from build123d import *

# Parameters (mm, degrees)
EXTRUDE_1_DEPTH     = 40
SKETCH_8_R          = 2
CUT_EXTRUDE_1_DEPTH = 50
SKETCH_9_R          = 2
CUT_EXTRUDE_2_DEPTH = 30
SKETCH_10_R         = 4.000599978
SKETCH_10_R_2       = 4
CUT_EXTRUDE_3_DEPTH = 10
CUT_EXTRUDE_START   = -10
SKETCH_11_R         = 4
CUT_EXTRUDE_4_DEPTH = 10
SKETCH_12_R         = 2
CUT_EXTRUDE_5_DEPTH = 40


with BuildPart() as part:
    # Эскиз1 → Бобышка-Вытянуть1 (new body)
    with BuildSketch(Plane.XY):
        with BuildLine():
            Line((0, 0), (130, 0))
            Line((130, 0), (130, 40))
            Line((130, 40), (0, 40))
            Line((0, 40), (0, 21))
            Line((0, 21), (12.566965626, 21))
            ThreePointArc((12.566965626, 21), (27.5, 20), (12.566965626, 19))
            Line((12.566965626, 19), (0, 19))
            Line((0, 19), (0, 0))
        make_face()
        with BuildLine():
            Line((67.433034374, 21), (77.433034374, 21))
            Line((77.433034374, 21), (77.433034374, 19))
            Line((77.433034374, 19), (67.433034374, 19))
            ThreePointArc((67.433034374, 19), (60, 12.5), (52.566965626, 19))
            Line((52.566965626, 19), (37.566965626, 19))
            Line((37.566965626, 19), (37.566965626, 21))
            Line((37.566965626, 21), (52.566965626, 21))
            ThreePointArc((52.566965626, 21), (60, 27.5), (67.433034374, 21))
        make_face(mode=Mode.SUBTRACT)
    extrude(amount=EXTRUDE_1_DEPTH)

    # Эскиз8 → Вырез-Вытянуть1 (cut)
    with BuildSketch(Plane.XZ):
        with Locations(Location((8, 30, 0), (0, 0, 270))):
            Circle(SKETCH_8_R)
        with Locations(Location((8, 10, 0), (0, 0, 270))):
            Circle(SKETCH_8_R)
        with Locations(Location((48, 30, 0), (0, 0, 270))):
            Circle(SKETCH_8_R)
        with Locations(Location((48, 10, 0), (0, 0, 270))):
            Circle(SKETCH_8_R)
    extrude(amount=-CUT_EXTRUDE_1_DEPTH, mode=Mode.SUBTRACT)

    # Эскиз9 → Вырез-Вытянуть2 (cut)
    with BuildSketch(Plane(origin=(130, 0, 0), x_dir=(0, 0, -1), z_dir=(1, 0, 0))):
        with Locations((-32, 35)):
            Circle(SKETCH_9_R)
        with Locations((-8, 35)):
            Circle(SKETCH_9_R)
        with Locations((-8, 5)):
            Circle(SKETCH_9_R)
        with Locations((-32, 5)):
            Circle(SKETCH_9_R)
    extrude(amount=-CUT_EXTRUDE_2_DEPTH, mode=Mode.SUBTRACT)

    # Эскиз10 → Вырез-Вытянуть3 (cut)
    with BuildSketch(Plane(origin=(0, 40, 0), x_dir=(1, 0, 0), z_dir=(0, 1, 0))):
        with Locations(Location((110, -8, 0), (0, 0, 270))):
            Circle(SKETCH_10_R)
        with Locations(Location((110, -32, 0), (0, 0, 270))):
            Circle(SKETCH_10_R_2)
    extrude(amount=-CUT_EXTRUDE_3_DEPTH, mode=Mode.SUBTRACT)

    # Эскиз11 → Вырез-Вытянуть4 (cut)
    with BuildSketch(Plane.XZ.offset(CUT_EXTRUDE_START)):
        with Locations(Location((110, 32, 0), (0, 0, 90))):
            Circle(SKETCH_11_R)
        with Locations(Location((110, 8, 0), (0, 0, 270))):
            Circle(SKETCH_11_R)
    extrude(amount=CUT_EXTRUDE_4_DEPTH, mode=Mode.SUBTRACT)

    # Эскиз12 → Вырез-Вытянуть5 (cut)
    with BuildSketch(Plane.XZ):
        with Locations(Location((72, 19, 0), (0, 0, 270))):
            Circle(SKETCH_12_R)
    extrude(amount=-CUT_EXTRUDE_5_DEPTH, mode=Mode.SUBTRACT)


solid = part.part
Could you check a few things on this model? Use its own coordinates, in mm. A direction names the side the tool comes from. Coordinates: 2 decimals unless noted, no trailing zeros. Write each loop counter-clockwise with the first axis right and the second up, starting at its lowest first coordinate (ties: lowest second). Pieces come first, ordered by that corner, then holes. Notation, with made-up numbers: M -35.75,-34.5 L 11.25,-34.5 A28 ccw 11.25,-3.5 Z; hole C 39.25,44 d7. An arc over 180 degrees is marked long. One line per question, with ' | ' between items.
1) I need wall thicknesses on probe 1 along Z at (x, y) = (101.75, 5); probe 2 along Y at (x, z) = (102.5, 8); probe 3 along Y at (x, z) = (19.5, 24.5). Which ranges of each line are inside material? Lowest first, please. Write a range as [from, to].
Checks:
probe 1: [0, 6], [10, 30], [34, 40] | probe 2: [0, 3], [7, 33], [37, 40] | probe 3: [0, 12.52], [27.48, 40]
2) Imagine slicing it at A-A, the plane x = 72. Write out the boundary of the cut face in (y, z), and give its area (3 significant figures).
Checks:
outline: M 0,0 L 19,0 L 19,17 L 0,17 Z; M 0,21 L 19,21 L 19,40 L 0,40 Z; M 21,0 L 40,0 L 40,17 L 21,17 Z; M 21,21 L 40,21 L 40,40 L 21,40 Z | area: 1,370 mm²
3) Imagine slicing it at D-D, the plane x = 48. Write out the boundary of the cut face in (y, z).
Checks:
outline: M 0,0 L 19,0 L 19,8 L 0,8 Z; M 0,12 L 19,12 L 19,28 L 0,28 Z; M 0,32 L 19,32 L 19,40 L 0,40 Z; M 21,0 L 40,0 L 40,8 L 21,8 Z; M 21,12 L 40,12 L 40,28 L 21,28 Z; M 21,32 L 40,32 L 40,40 L 21,40 Z
4) Imagine slicing it at C-C, the plane z = 37.5. Write out the boundary of the cut face in (x, y), and give its area (3 significant figures).
Checks:
outline: M 0,0 L 130,0 L 130,40 L 0,40 L 0,21 L 12.57,21 A7.5 cw long 12.57,19 L 0,19 Z; hole M 37.57,19 L 52.57,19 A7.5 ccw 67.43,19 L 77.43,19 L 77.43,21 L 67.43,21 A7.5 ccw 52.57,21 L 37.57,21 Z | area: 4,770 mm²
5) For pin 1 Ø2.5 at (x, z) = (111, 9.5) entering from +Y; pin 2 Ø1.2 at (y, z) = (34.5, 7.5) entering from +X; pin 3 Ø3.5 at (x, z) = (48, 30) entering from +Y, each with a flat end and sliding along its axis, tell me the tip position at first contact or that it passes through.
Checks:
pin 1: y = 30 | pin 2: x = 100 | pin 3: through
6) For faces 1 (the face through (10, 30, 10)), 2 (the face through (100, 5, 8)), 3 (the face through (113.373, 5.07, 5.85)), 4 (the face through (110, 30, 8)), 5 (the face through (75, 21, 20)), which set-ups out of +Z, -Z, +X, -X, +Y, -Y let a thin tool reach every point of the face, with its end or its side?
Checks:
face 1: +Y, -Y | face 2: +X | face 3: -Y | face 4: +Y | face 5: +Z, -Z
7) If we mould it in two halves opening along Y, with no side actions, what happens to faces 6 (the face through (100, 35, 8)), 7 (the face through (8.601, 9.367, 28.092)), 8 (the face through (75, 19, 20)), 9 (the face through (110, 10, 8))? For each: released by +Y, released by -Y, zero draft, split by the parting line, or undercut.
Checks:
face 6: undercut | face 7: zero draft | face 8: undercut | face 9: released by -Y
8) Imagine slicing it at B-B, the plane y = 24. Write out the boundary of the cut face in (x, z).
Checks:
outline: M 0,0 L 13.66,0 L 13.66,40 L 0,40 Z; M 26.34,0 L 53.66,0 L 53.66,40 L 26.34,40 Z; M 66.34,0 L 130,0 L 130,40 L 66.34,40 Z; hole C 8,10 d4; hole C 8,30 d4; hole C 48,10 d4; hole C 48,30 d4; hole C 72,19 d4
